Autodesk Inventor part; units mm, degrees
ref_plane "YZ Plane" through (0, 0, 0) normal (1, 0, 0) x (0, 1, 0)
ref_plane "XZ Plane" through (0, 0, 0) normal (0, 1, 0) x (-1, 0, 0)
ref_plane "XY Plane" through (0, 0, 0) normal (0, 0, 1) x (1, 0, 0)
ref_plane "Arbeitsebene1" through (-23.7843, -50.4597, 67.3862) normal (0, -1, 0) x (-1, 0, 0)
sketch "Skizze1" plane through (-23.7843, -50.4597, 67.3862) normal (0, -1, 0) x (-1, 0, 0)
  arc A0 (-13.7675, -44.4592) -> (52.565, -44.4592) centre (19.3987, 5.5408) ccw
  arc A1 (52.565, -44.4592) -> (-13.7675, -44.4592) centre (19.3987, -94.4592) ccw
  arc A2 (-12.8526, -43.8642) -> (51.65, -43.8642) centre (19.3987, 5.5408) ccw
  arc A3 (51.65, -45.0542) -> (-12.8526, -45.0542) centre (19.3987, -94.4592) ccw
  line L0 (30.3074, -55.4592) -> (8.49, -55.4592)
  line L1 (8.49, -55.4592) -> (8.49, -53.4592)
  line L2 (8.49, -53.4592) -> (30.3074, -53.4592)
  line L3 (30.3074, -53.4592) -> (30.3074, -55.4592)
  line L4 (30.3074, -55.4592) -> (8.49, -53.4592) construction
  line L5 (8.49, -55.4592) -> (30.3074, -53.4592) construction
  point P0 (-23.7843, 67.3862)
  point P1 (50.7196, -44.4592)
  point P2 (-11.9222, -44.4592)
  point P3 (19.3987, -54.4592)
  dimension "d0" = 120
  dimension "d1" = 120
  dimension "d2" = 100
  dimension "d3" = 0
  dimension "d4" = 1
  dimension "d5" = 1
extrude "Extrusion1" add sketch "Skizze1" along normal blind 20 contours A1 A2 A3 A0 | A3 A2 L2 A0 | A1 A2 A3 | L2 A0 | A0 L3 L0 L1 | A1 A0 A3 A2 | L2 A2 A3 A0
properties part number "07_Feder"
CAD build for the part. Positions are in the model's coordinates, mm. Coordinates: 2 decimals unless noted, no trailing zeros. Order: outer loops, then holes, each group sorted by start corner. A loop starts at its lowest first (then second) coordinate and runs counter-clockwise, first axis right, second up. Notation, with made-up numbers: (-21.75, 58.5) - (-8.75, 58.5) arc R27 cw to (-8.75, 90.5) - close; hole circle Ø8 at (39.5, -8.75). An arc over 180 degrees is marked (long way). Answer in a Markdown table with one row per item.
1. Flat gauge pins, fed straight in: P1, Ø10, axis at x = -30.5, y = -61.5, coming from the -Z side; P2, Ø3, axis at x = -40, y = -65, coming from the -Z side; P3, Ø2, axis at y = -59, z = 122, coming from the -X side. Where does each tip first touch, or does it go through?
Answer:
| item | result |
|---|---|
| P1 | z = 102.34 |
| P2 | z = 101.87 |
| P3 | x = -54.09 |
2. Slice it at A-A, the plane y = -67. List the corners of the cut face in (x, z), then the cut area to 3 significant figures.
Answer:
| item | result |
|---|---|
| outline | (-76.35, 111.85) arc R60 ccw to (-10.02, 111.85) arc R60 ccw to (-32.27, 120.85) - (-32.27, 122.85) - (-54.09, 122.85) - (-54.09, 120.85) arc R60 ccw to start; hole (-74.5, 111.85) arc R59 ccw to (-11.86, 111.85) arc R59 ccw to start |
| area | 165 mm² |
3. Pull direction Z, two halves, no side cores. Call faces 1 (the face through (-32.274, -60, 122)), 2 (the face through (-43, -60, 122.845)), 3 (the face through (-42.721, -60.32, 102.847)): +Z half, -Z half, draft (parallel to the pull), parting line (faces both ways), or undercut.
Answer:
| item | result |
|---|---|
| face 1 | draft |
| face 2 | +Z half |
| face 3 | undercut |
4. Slice it at C-C, the plane x = -59. List the corners of the cut face in (y, z), then the cut area to 3 significant figures.
Answer:
| item | result |
|---|---|
| outline | (-70.46, 103.97) - (-50.46, 103.97) - (-50.46, 105.01) - (-70.46, 105.01) - close; (-70.46, 118.69) - (-50.46, 118.69) - (-50.46, 119.72) - (-70.46, 119.72) - close |
| area | 41.5 mm² |
5. Slice it at B-B, the plane z = 105.5. List the corners of the cut face in (x, y), then the cut area to 3 significant figures.
Answer:
| item | result |
|---|---|
| outline | (-63.8, -70.46) - (-60.68, -70.46) - (-60.68, -50.46) - (-63.8, -50.46) - close; (-25.68, -70.46) - (-22.56, -70.46) - (-22.56, -50.46) - (-25.68, -50.46) - close |
| area | 125 mm² |
6. Drill centre lines: L1, parallel to X at y = -55.75, z = 122; L2, parallel to X at y = -69.5, z = 114.25; L3, parallel to Z at x = -51, y = -51.5. Where is each one in solid material? Low to high. Write a range as from..to.
Answer:
| item | result |
|---|---|
| L1 | -54.09..-32.27 |
| L2 | -72.4..-70.29, -16.08..-13.96 |
| L3 | 102.36..103.37, 120.33..122.85 |
